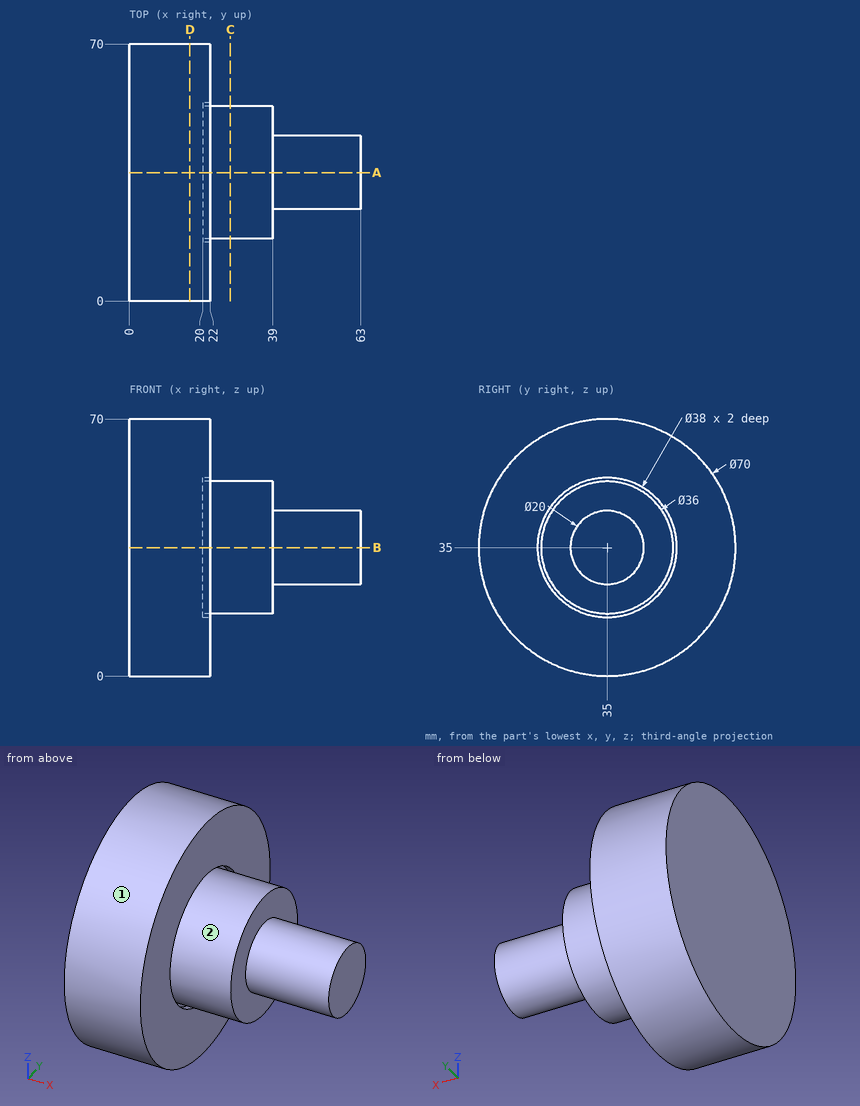
Input: dimensioned drawing with shaded views. Units: mm. Origin: part minimum x, y, z. A direction names the side the tool comes from. Coordinates: 2 decimals unless noted, no trailing zeros. Loops run counter-clockwise (first coordinate to the right, second up) from the corner with the lowest first, then second, coordinate; pieces in that order, holes last. Notation, with made-up numbers: M -2.5,32 L 6.5,32 A34 ccw 6.5,71 Z; hole C -39.75,46.25 d3. An arc over 180 degrees is marked long. One line per item, written item: value. Start each with the question number.
1) Reachability of the marked faces 1 and 2 from +Z, -Z, +X, -X, +Y, -Y: full face, straight path, thin tool, end or side. Return the list, or none.
2) Cut plane C-C (x = 27.5). Return loops of the section in (y, z), then the cut area to 3 significant figures.
3) Material intervals for L1, parallel to Y at x = 20.8, z = 35; L2, parallel to X at y = 24.5, z = 50; L3, parallel to X at y = 33, z = 63, sorted ascending. Write a range as from..to.
4) Cut plane D-D (x = 16.5). Return loops of the section in (y, z).
5) Cut plane A-A (y = 35). Return loops of the section in (x, z).
6) Pin query (flat end, axial travel): P1, Ø8, axis at x = 6.5, z = 11, coming from the +Y side; P2, Ø4, axis at x = 43.5, y = 45.5, coming from the -Z side; P3, Ø3, axis at x = 48.5, z = 29, coming from the +Y side. Return the tip coordinate at first contact, or that it passes through.
Evaluation:
1. face 1: +X, -X
1. face 2: +X
2. outline: C 35,35 d36
2. area: 1,020 mm^2
3. L1: 0..16, 17..53, 54..70
3. L2: 0..20
3. L3: 0..22
4. outline: C 35,35 d70
5. outline: M 0,0 L 22,0 L 22,16 L 20,16 L 20,17 L 39,17 L 39,25 L 63,25 L 63,45 L 39,45 L 39,53 L 20,53 L 20,54 L 22,54 L 22,70 L 0,70 Z
6. P1: y = 63.72
6. P2: z = 29.73
6. P3: y = 43.93
